Here's how the part is built. I have some questions about the finished solid (model axes, mm). A direction names the side the tool comes from. Round coordinates to 2 decimals unless told otherwise and drop trailing zeros. Write each loop counter-clockwise with the first axis right and the second up, starting at its lowest first coordinate (ties: lowest second). Pieces come first, ordered by that corner, then holes. Notation, with made-up numbers: (48, -7) - (92, -7) arc R16 ccw to (92, 20) - close; hole circle Ø9 at (-39, 54.25). An arc over 180 degrees is marked (long way). One line per question, with ' | ' between items. Start each with the question number.
(1) Thinking about a two-plate mould opening in Y: for faces 4 (the flat face through (471, -28, 75)), 5 (the flat face through (493, 0, 18)), 6 (the cylindrical face through (535.993, -0.616, 27.367)), 7 (the cylindrical face through (520.4, 3.9, 77.4)), which applies, pulls with the +Y half, pulls with the -Y half, needs draft (parallel to the pull), parting line crosses it, or undercut?
(2) Imagine slicing it at C-C (x = 363). Write out the boundary of the cut face in (y, z).
(3) Imagine slicing it at A-A (z = 31). Write out the boundary of the cut face in (x, y).
(4) If I drill on L1, parallel to Y at x = 508, z = 72.5; L2, parallel to Z at x = 495, y = 14; L3, parallel to X at y = 0, z = 75, over which ranges is the centre line in solid material (lowest first)?
(5) Will these pins go through, and if not, where does the flat tip stop? pin 1 (9 mm diameter, centred on y = 1, z = 98.5, fed in from +X); pin 2 (5 mm diameter, centred on y = 5.5, z = 35.5, fed in from +X); pin 3 (8 mm diameter, centred on y = -23.5, z = 56.5, fed in from -X); pin 4 (23.5 mm diameter, centred on x = 508, y = 0, fed in from -Z).
(6) Imagine slicing it at D-D (y = -15.5). Write out the boundary of the cut face in (x, z).
(7) Imagine slicing it at B-B (y = 2.5). Write out the boundary of the cut face in (x, z).
(8) For faces 1 (the flat face through (451.129, 0, 9)), 2 (the flat face through (447.429, -20, 52)), 3 (the flat face through (359, 12.5, 52)), which set-ups out of +Z, -Z, +X, -X, +Y, -Y let a thin tool reach every point of the face, with its end or its side?
from build123d import *

# Parameters (mm, degrees)
F0_R     = 13
F1_DEPTH = 105
F3_DEPTH = 52.5


with BuildPart() as f1:
    # F0 (on Top) → F1 (new body)
    with BuildSketch(Plane.XY):
        with BuildLine():
            Line((447.4289454073, -28), (508, -28))
            ThreePointArc((508, -28), (536, 0), (508, 28))
            Line((508, 28), (447.4289454073, 28))
            Line((447.4289454073, 28), (447.4289454073, 12.5))
            Line((447.4289454073, 12.5), (218.8289454073, 12.5))
            Line((218.8289454073, 12.5), (218.8289454073, -12.5))
            Line((218.8289454073, -12.5), (447.4289454073, -12.5))
            Line((447.4289454073, -12.5), (447.4289454073, -28))
        make_face()
        with Locations((508, 0)):
            Circle(F0_R, mode=Mode.SUBTRACT)
    extrude(amount=F1_DEPTH)


with BuildPart() as f3:
    # F2 (on Front) → F3 (new body, symmetric)
    with BuildSketch(Plane.XZ):
        Polygon((268.3927469848, 105), (268.3927469848, 0), (451.1286479985, 0), (451.1286479985, 18), (537.2693231227, 18), (537.2693231227, 37), (451.1286479985, 37), (451.1286479985, 68), (537.2693231227, 68), (537.2693231227, 87), (451.1286479985, 87), (451.1286479985, 105), align=None)
    extrude(amount=F3_DEPTH, both=True)


with BuildPart() as f1_1:
    add(f1.part)

    # F4: intersect F3
    add(f3.part, mode=Mode.INTERSECT)


solid = f1_1.part
Check sheet entries:
1) face 4: pulls with the -Y half | face 5: needs draft | face 6: parting line crosses it | face 7: undercut
2) outline: (-12.5, 0) - (12.5, 0) - (12.5, 105) - (-12.5, 105) - close
3) outline: (268.39, -12.5) - (447.43, -12.5) - (447.43, -28) - (508, -28) arc R28 ccw to (508, 28) - (447.43, 28) - (447.43, 12.5) - (268.39, 12.5) - close; hole circle Ø26 at (508, 0)
4) L1: -28 to -13, 13 to 28 | L2: 18 to 37, 68 to 87 | L3: 268.39 to 495, 521 to 536
5) pin 1: x = 451.13 | pin 2: x = 535.84 | pin 3: x = 447.43 | pin 4: through
6) outline: (447.43, 0) - (451.13, 0) - (451.13, 18) - (531.32, 18) - (531.32, 37) - (451.13, 37) - (451.13, 68) - (531.32, 68) - (531.32, 87) - (451.13, 87) - (451.13, 105) - (447.43, 105) - close
7) outline: (268.39, 0) - (451.13, 0) - (451.13, 18) - (495.24, 18) - (495.24, 37) - (451.13, 37) - (451.13, 68) - (495.24, 68) - (495.24, 87) - (451.13, 87) - (451.13, 105) - (268.39, 105) - close; (520.76, 18) - (535.89, 18) - (535.89, 37) - (520.76, 37) - close; (520.76, 68) - (535.89, 68) - (535.89, 87) - (520.76, 87) - close
8) face 1: -Z, +X, +Y, -Y | face 2: +Z, -Z, -X, -Y | face 3: +Z, -Z, -X, +Y
